from build123d import *

# Parameters (mm, degrees)
F0_W            = 30
F0_H            = 30
F1_DEPTH        = 30
F2_T            = -2.5
F6_DEPTH        = 10.5
F9_DEPTH        = 10.5
F11_DEPTH       = 4.5
F12_DEPTH       = 4.5
F14_D           = 2
F14_DEPTH       = 15
F14_CBORE_D     = 5
F14_CBORE_DEPTH = 0.9
F14_TIP         = 0.600860619
F15_R           = 4
F15_R_2         = 1.5
F16_DEPTH       = 10.5


with BuildPart() as f1:
    # F0 (on Top) → F1 (new body)
    with BuildSketch(Plane.XY):
        Rectangle(F0_W, F0_H)
    extrude(amount=F1_DEPTH)

    # F2 (hollow: no face is removed)
    offset(amount=F2_T, mode=Mode.SUBTRACT)

    # F3 (on Top) → F6 (join, through all)
    with BuildSketch(Plane.XY):
        with BuildLine():
            ThreePointArc((3.75, 6.4951905284), (6.4951905284, 3.75), (7.5, 0))
            ThreePointArc((7.5, 0), (6.4951905284, -3.75), (3.75, -6.4951905284))
            Line((3.75, -6.4951905284), (3.75, -12.5))
            Line((3.75, -12.5), (12.5, -12.5))
            Line((12.5, -12.5), (12.5, 12.5))
            Line((12.5, 12.5), (3.75, 12.5))
            Line((3.75, 12.5), (3.75, 6.4951905284))
        make_face()
        with BuildLine():
            Line((-3.75, 6.4951905284), (-3.75, 12.5))
            Line((-3.75, 12.5), (-12.5, 12.5))
            Line((-12.5, 12.5), (-12.5, -12.5))
            Line((-12.5, -12.5), (-3.75, -12.5))
            Line((-3.75, -12.5), (-3.75, -6.4951905284))
            ThreePointArc((-3.75, -6.4951905284), (-6.4951905284, -3.75), (-7.5, 0))
            ThreePointArc((-7.5, 0), (-6.4951905284, 3.75), (-3.75, 6.4951905284))
        make_face()
    extrude(amount=F6_DEPTH)

    # F7 (on face) → F9 (join, through all)
    with BuildSketch(Plane.XY.offset(30)):
        with BuildLine():
            ThreePointArc((3.75, 6.4951905284), (6.4951905284, 3.75), (7.5, 0))
            ThreePointArc((7.5, 0), (6.4951905284, -3.75), (3.75, -6.4951905284))
            Line((3.75, -6.4951905284), (3.75, -12.5))
            Line((3.75, -12.5), (12.5, -12.5))
            Line((12.5, -12.5), (12.5, 12.5))
            Line((12.5, 12.5), (3.75, 12.5))
            Line((3.75, 12.5), (3.75, 6.4951905284))
        make_face()
        with BuildLine():
            Line((-3.75, 6.4951905284), (-3.75, 12.5))
            Line((-3.75, 12.5), (-12.5, 12.5))
            Line((-12.5, 12.5), (-12.5, -12.5))
            Line((-12.5, -12.5), (-3.75, -12.5))
            Line((-3.75, -12.5), (-3.75, -6.4951905284))
            ThreePointArc((-3.75, -6.4951905284), (-6.4951905284, -3.75), (-7.5, 0))
            ThreePointArc((-7.5, 0), (-6.4951905284, 3.75), (-3.75, 6.4951905284))
        make_face()
    extrude(amount=-F9_DEPTH)

    # F10 (on mid) → F11 (join, through all)
    with BuildSketch(Plane.XY.offset(15)):
        with BuildLine():
            Line((3.75, -10.6066017178), (3.75, -12.5))
            Line((3.75, -12.5), (12.5, -12.5))
            Line((12.5, -12.5), (12.5, 12.5))
            Line((12.5, 12.5), (3.75, 12.5))
            Line((3.75, 12.5), (3.75, 10.6066017178))
            ThreePointArc((3.75, 10.6066017178), (11.25, 0), (3.75, -10.6066017178))
        make_face()
        with BuildLine():
            Line((-3.75, 10.6066017178), (-3.75, 12.5))
            Line((-3.75, 12.5), (-12.5, 12.5))
            Line((-12.5, 12.5), (-12.5, -12.5))
            Line((-12.5, -12.5), (-3.75, -12.5))
            Line((-3.75, -12.5), (-3.75, -10.6066017178))
            ThreePointArc((-3.75, -10.6066017178), (-11.25, 0), (-3.75, 10.6066017178))
        make_face()
    extrude(amount=-F11_DEPTH)

    # F10 (on mid) → F12 (join, through all)
    with BuildSketch(Plane.XY.offset(15)):
        with BuildLine():
            Line((3.75, -10.6066017178), (3.75, -12.5))
            Line((3.75, -12.5), (12.5, -12.5))
            Line((12.5, -12.5), (12.5, 12.5))
            Line((12.5, 12.5), (3.75, 12.5))
            Line((3.75, 12.5), (3.75, 10.6066017178))
            ThreePointArc((3.75, 10.6066017178), (11.25, 0), (3.75, -10.6066017178))
        make_face()
        with BuildLine():
            Line((-3.75, 10.6066017178), (-3.75, 12.5))
            Line((-3.75, 12.5), (-12.5, 12.5))
            Line((-12.5, 12.5), (-12.5, -12.5))
            Line((-12.5, -12.5), (-3.75, -12.5))
            Line((-3.75, -12.5), (-3.75, -10.6066017178))
            ThreePointArc((-3.75, -10.6066017178), (-11.25, 0), (-3.75, 10.6066017178))
        make_face()
    extrude(amount=F12_DEPTH)

    # F14
    with Locations(Plane.YZ.offset(15)):
        with Locations((0, 5), (0, 25)):
            CounterBoreHole(F14_D / 2, F14_CBORE_D / 2, F14_CBORE_DEPTH, depth=F14_DEPTH)
            with Locations((0, 0, -(F14_DEPTH + F14_TIP / 2))):  # 118° drill point
                Cone(0, F14_D / 2, F14_TIP, mode=Mode.SUBTRACT)

    # F15 (on Top) → F16 (join, through all)
    with BuildSketch(Plane.XY):
        Circle(F15_R)
        Circle(F15_R_2, mode=Mode.SUBTRACT)
    extrude(amount=F16_DEPTH)


solid = f1.part
Verification items for the finished model (mm, model axes). A direction names the side the tool comes from. Coordinates: 2 decimals unless noted, no trailing zeros. Order: outer loops, then holes, each group sorted by start corner. A loop starts at its lowest first (then second) coordinate and runs counter-clockwise, first axis right, second up.
1. Sectioned sample at D-D, the plane y = -6. Record the cut outline in (x, z).
Results found:
outline: (-15, 0) - (15, 0) - (15, 30) - (-15, 30) - close; hole (-9.52, 10.5) - (-4.5, 10.5) - (-4.5, 2.5) - (4.5, 2.5) - (4.5, 10.5) - (9.52, 10.5) - (9.52, 19.5) - (4.5, 19.5) - (4.5, 27.5) - (-4.5, 27.5) - (-4.5, 19.5) - (-9.52, 19.5) - close
2. Set-up check for faces 1 (the face through (11, 0, 6)), 2 (the face through (15, 0, 15)), 3 (the face through (0, 0, 27.5)): record each of +Z, -Z, +X, -X, +Y, -Y from which the full face is reachable in a straight line by a thin tool's end or side.
Results found:
face 1: +X
face 2: +Z, -Z, +X, +Y, -Y
face 3: none
3. Sectioned sample at B-B, the plane z = 9.75. Record the cut outline in (x, y), and give its area (3 significant figures).
Results found:
outline: (-15, -15) - (15, -15) - (15, 15) - (-15, 15) - close; circle Ø8 at (0, 0); hole (-3.75, -12.5) - (3.75, -12.5) - (3.75, -6.5) arc R7.5 ccw to (3.75, 6.5) - (3.75, 12.5) - (-3.75, 12.5) - (-3.75, 6.5) arc R7.5 ccw to (-3.75, -6.5) - close; hole circle Ø3 at (0, 0)
area: 687 mm2
4. Sectioned sample at C-C, the plane x = 0. Record the cut outline in (y, z), and give its area (3 significant figures).
Results found:
outline: (-15, 0) - (15, 0) - (15, 30) - (-15, 30) - close; hole (-12.5, 2.5) - (-4, 2.5) - (-4, 10.5) - (-1.5, 10.5) - (-1.5, 2.5) - (1.5, 2.5) - (1.5, 10.5) - (4, 10.5) - (4, 2.5) - (12.5, 2.5) - (12.5, 27.5) - (-12.5, 27.5) - close
area: 315 mm2
5. Release check for a two-part mould opening along Z. For faces 4 (the face through (0, 0, 0)), 5 (the face through (-8, 0, 10.5)), 6 (the face through (0, 15, 15)) record: +Z half, -Z half, draft (parallel to the pull), parting line (faces both ways), or undercut.
Results found:
face 4: -Z half
face 5: undercut
face 6: draft
6. Scan lines: line 1 (Z direction, x = 11.5, y = 0); line 2 (Y direction, x = 0, z = 6.5); line 3 (X direction, y = -12, z = 4.75). Record each from-to range of solid material in increasing order.
Results found:
line 1: z = 0 to 4, 6 to 24, 26 to 30
line 2: y = -15 to -12.5, -4 to -1.5, 1.5 to 4, 12.5 to 15
line 3: x = -15 to -3.75, 3.75 to 15
7. Sectioned sample at A-A, the plane z = 5. Record the cut outline in (x, y).
Results found:
outline: (-15, -15) - (15, -15) - (15, -2.5) - (14.1, -2.5) - (14.1, -1) - (7.43, -1) arc R7.5 cw to (3.75, -6.5) - (3.75, -12.5) - (-3.75, -12.5) - (-3.75, -6.5) arc R7.5 cw to (-3.75, 6.5) - (-3.75, 12.5) - (3.75, 12.5) - (3.75, 6.5) arc R7.5 cw to (7.43, 1) - (14.1, 1) - (14.1, 2.5) - (15, 2.5) - (15, 15) - (-15, 15) - close; circle Ø8 at (0, 0); hole circle Ø3 at (0, 0)
